Read the model definition and answer for the solid it produces. Units are mm, in the model's axes. Face numbers are marked on the shaded views. Coordinates: 2 decimals unless noted, no trailing zeros. Order: outer loops, then holes, each group sorted by start corner. A loop starts at its lowest first (then second) coordinate and runs counter-clockwise, first axis right, second up. Notation, with made-up numbers: (-31.75, 56.5) -> (-26.75, 56.5) arc R20 ccw to (-26.75, 79.5) -> close; hole circle Ø5 at (64.25, 83). An arc over 180 degrees is marked (long way). Use CSV: the item, a comma, the result in double quotes.
```python
from build123d import *

# Parameters (mm, degrees)
SKETCH1_W           = 33.8709
SKETCH1_H           = 38.1
BOSS_EXTRUDE1_DEPTH = 1.599999848
SKETCH2_W           = 26.4795
SKETCH2_H           = 36.4998
SKETCH2_W_2         = 25.5795
SKETCH2_H_2         = 35.5998
BOSS_EXTRUDE2_DEPTH = 1.4
SKETCH3_W           = 12.7
SKETCH3_H           = 38.1
BOSS_EXTRUDE3_DEPTH = 1.5875


with BuildPart() as part:
    # Sketch1 → Boss-Extrude1 (new body)
    with BuildSketch(Plane.XY):
        Rectangle(SKETCH1_W, SKETCH1_H)
    extrude(amount=BOSS_EXTRUDE1_DEPTH)

    # Sketch2 → Boss-Extrude2 (add)
    with BuildSketch(Plane.XY.offset(1.599999848)):
        with Locations((-2.1082, 0)):
            Rectangle(SKETCH2_W, SKETCH2_H)
        with Locations((-2.1082, 0)):
            Rectangle(SKETCH2_W_2, SKETCH2_H_2, mode=Mode.SUBTRACT)
    extrude(amount=BOSS_EXTRUDE2_DEPTH)

    # Sketch3 → Boss-Extrude3 (add)
    with BuildSketch(Plane(origin=(16.93545, 0, 0), x_dir=(0, 0, -1), z_dir=(1, 0, 0))):
        with Locations((-6.35, 0)):
            Rectangle(SKETCH3_W, SKETCH3_H)
    extrude(amount=BOSS_EXTRUDE3_DEPTH)


solid = part.part
```
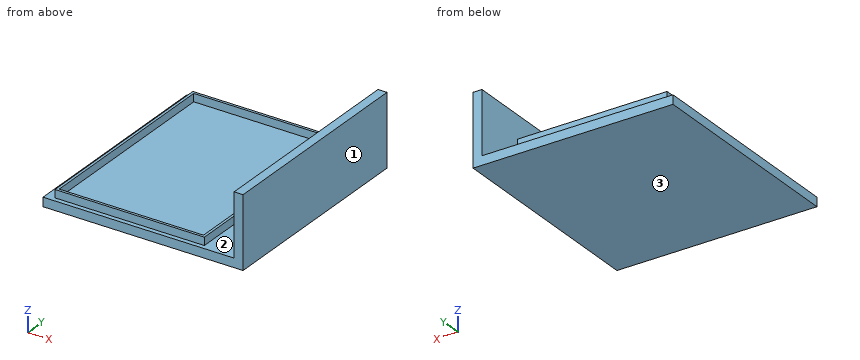
Item 1: Find section C-C, the plane z = 3.5. Give the vertices of the cut face in (x, y), then the cut area to 3 significant figures.
Return value:
outline,"(16.94, -19.05) -> (18.52, -19.05) -> (18.52, 19.05) -> (16.94, 19.05) -> close"
area,"60.5 mm^2"
Item 2: Find section A-A, the plane y = -13.5. Give the vertices of the cut face in (x, z).
Return value:
outline,"(-16.94, 0) -> (18.52, 0) -> (18.52, 12.7) -> (16.94, 12.7) -> (16.94, 1.6) -> (11.13, 1.6) -> (11.13, 3) -> (10.68, 3) -> (10.68, 1.6) -> (-14.9, 1.6) -> (-14.9, 3) -> (-15.35, 3) -> (-15.35, 1.6) -> (-16.94, 1.6) -> close"
Item 3: Each of these flat-tipped pins is pushed along its axis until it touches: P1, Ø0.7, axis at x = -5, z = 2.5, coming from the +Y side; P2, Ø13, axis at x = 3.5, y = -2, coming from the +Z side; P3, Ø1, axis at x = 6, z = 5, coming from the -Y side; P4, Ø0.7, axis at x = -8.5, z = 2.5, coming from the -Y side. Where does it stop, or does it pass through?
Return value:
P1,"stops at y = 18.25"
P2,"stops at z = 1.6"
P3,"passes through"
P4,"stops at y = -18.25"
Item 4: Find section B-B, the plane x = 5. Give the vertices of the cut face in (y, z).
Return value:
outline,"(-19.05, 0) -> (19.05, 0) -> (19.05, 1.6) -> (18.25, 1.6) -> (18.25, 3) -> (17.8, 3) -> (17.8, 1.6) -> (-17.8, 1.6) -> (-17.8, 3) -> (-18.25, 3) -> (-18.25, 1.6) -> (-19.05, 1.6) -> close"
Item 5: Find section D-D, the plane x = 12.5. Give the vertices of the cut face in (y, z).
Return value:
outline,"(-19.05, 0) -> (19.05, 0) -> (19.05, 1.6) -> (-19.05, 1.6) -> close"
Item 6: The mould has two halves that part along X. Classify the marked faces 1, 2 and 3: +X half, -X half, draft (parallel to the pull), parting line (faces both ways), or undercut.
Return value:
face 1,"+X half"
face 2,"undercut"
face 3,"draft"
Item 7: Straight lines are drawn through the part: line 1 along X through (y, z) = (-16, 2.5); line 2 along Y through (x, z) = (3, 2.5); line 3 along Z through (x, y) = (6.5, -16). For each, find the intervals that lie inside material, in ascending order.
Return value:
line 1,"x = -15.35 to -14.9, 10.68 to 11.13, 16.94 to 18.52"
line 2,"y = -18.25 to -17.8, 17.8 to 18.25"
line 3,"z = 0 to 1.6"
